The listing builds one solid part. Answer for the finished solid, in the listing's coordinates (mm). Round coordinates to 2 decimals unless told otherwise and drop trailing zeros. Loops run counter-clockwise (first coordinate to the right, second up) from the corner with the lowest first, then second, coordinate; pieces in that order, holes last. Notation, with made-up numbers: (10, 81.25) -> (32, 81.25) arc R23 cw to (32, 94.25) -> close; hole circle Ø9 at (41, 38). An arc over 180 degrees is marked (long way). Write each question's results on one line, items separated by ' | '. Start each with the question number.
from build123d import *

# Parameters (mm, degrees)
SKETCH_1_R      = 13.25
SKETCH_1_R_2    = 2
SKETCH_1_R_3    = 2.5
SKETCH_1_R_4    = 13
EXTRUDE_1_DEPTH = 5
FILLET_1_R      = 5


with BuildPart() as part:
    # 草图1 → 凸台-拉伸1 (new body)
    with BuildSketch(Plane.XY):
        with BuildLine():
            Line((0, 25), (124.869292101, 25))
            Line((124.869292101, 25), (184, 25))
            ThreePointArc((184, 25), (208.968890762, 1.246793543), (186.490484142, -24.875640469))
            Line((186.490484142, -24.875640469), (124.869292101, -25))
            Line((124.869292101, -25), (0, -25))
            Line((0, -25), (-16, -25))
            Line((-16, -25), (-16, 25))
            Line((-16, 25), (0, 25))
        make_face()
        with Locations((184, 0)):
            Circle(SKETCH_1_R, mode=Mode.SUBTRACT)
        with Locations((5, 16)):
            Circle(SKETCH_1_R_2, mode=Mode.SUBTRACT)
        with Locations(Location((5, -16, 0), (0, 0, 180))):
            Circle(SKETCH_1_R_2, mode=Mode.SUBTRACT)
        with Locations((60, 18)):
            Circle(SKETCH_1_R_3, mode=Mode.SUBTRACT)
        with Locations((124, 18)):
            Circle(SKETCH_1_R_3, mode=Mode.SUBTRACT)
        with Locations((34, 0)):
            Circle(SKETCH_1_R_4, mode=Mode.SUBTRACT)
        with Locations((34, 17.5)):
            Circle(SKETCH_1_R_2, mode=Mode.SUBTRACT)
        with Locations(Location((124, -18, 0), (0, 0, 180))):
            Circle(SKETCH_1_R_3, mode=Mode.SUBTRACT)
        with Locations(Location((60, -18, 0), (0, 0, 180))):
            Circle(SKETCH_1_R_3, mode=Mode.SUBTRACT)
        with Locations((51.5, 0)):
            Circle(SKETCH_1_R_2, mode=Mode.SUBTRACT)
        with Locations((34, -17.5)):
            Circle(SKETCH_1_R_2, mode=Mode.SUBTRACT)
        with Locations((16.5, 0)):
            Circle(SKETCH_1_R_2, mode=Mode.SUBTRACT)
        with Locations((-7, 16)):
            Circle(SKETCH_1_R_2, mode=Mode.SUBTRACT)
        with Locations(Location((-7, -16, 0), (0, 0, 180))):
            Circle(SKETCH_1_R_2, mode=Mode.SUBTRACT)
        with BuildLine():
            Line((75, -12), (110, -12))
            ThreePointArc((110, -12), (113, -9), (110, -6))
            Line((110, -6), (75, -6))
            ThreePointArc((75, -6), (72, -9), (75, -12))
        make_face(mode=Mode.SUBTRACT)
        with BuildLine():
            Line((124, 3), (159, 3))
            ThreePointArc((159, 3), (162, 0), (159, -3))
            Line((159, -3), (124, -3))
            ThreePointArc((124, -3), (121, 0), (124, 3))
        make_face(mode=Mode.SUBTRACT)
        with BuildLine():
            Line((75, 12), (110, 12))
            ThreePointArc((110, 12), (113, 9), (110, 6))
            Line((110, 6), (75, 6))
            ThreePointArc((75, 6), (72, 9), (75, 12))
        make_face(mode=Mode.SUBTRACT)
    extrude(amount=EXTRUDE_1_DEPTH)

    # 圆角1
    fillet_1_edges = [part.edges().sort_by_distance(p)[0] for p in [
        (-16, -25, 2.5),
        (-16, 25, 2.5),
    ]]
    fillet(fillet_1_edges, radius=FILLET_1_R)


solid = part.part
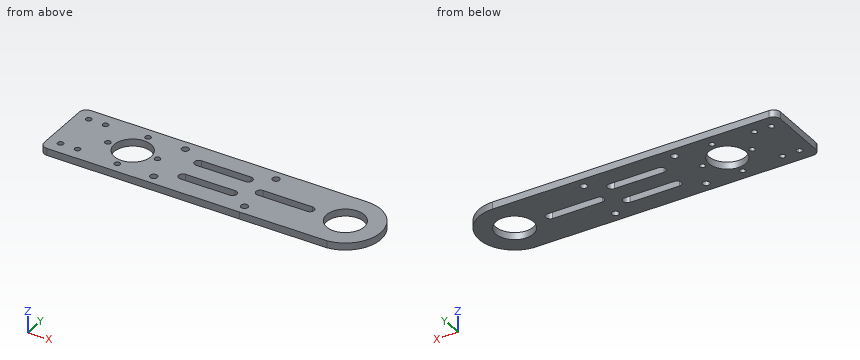
Item 1: The part is cut by section B-B, the plane x = 34. Give the vertices of the cut face in (y, z), plus the area to 3 significant figures.
Item 2: The part is cut by section A-A, the plane x = 5. Give the vertices of the cut face in (y, z), plus the area to 3 significant figures.
Item 3: Straight lines are drawn through the part: L1, parallel to Y at x = 5, z = 2; L2, parallel to Y at x = 110.5, z = 1.75; L3, parallel to X at y = 11, z = 1.95. For each, find the intervals that lie inside material, in ascending order. Write a range as [from, to].
Item 4: Each of these flat-tipped pins is pushed along its axis until it touches: pin 1 Ø3 at (x, z) = (139, 2) entering from -Y; pin 2 Ø2 at (y, z) = (-5, 1) entering from +X. Where does it stop, or does it pass through?
Item 5: The part is cut by section C-C, the plane y = 8.5. Give the vertices of the cut face in (x, z), plus the area to 3 significant figures.
Item 6: The part is cut by section D-D, the plane z = 3.2. Give the number of separate pieces and of enclosed holes in the cut face, plus the area to 3 significant figures.
Report:
1) outline: (-25, 0) -> (-19.5, 0) -> (-19.5, 5) -> (-25, 5) -> close; (-15.5, 0) -> (-13, 0) -> (-13, 5) -> (-15.5, 5) -> close; (13, 0) -> (15.5, 0) -> (15.5, 5) -> (13, 5) -> close; (19.5, 0) -> (25, 0) -> (25, 5) -> (19.5, 5) -> close | area: 80.0 mm2
2) outline: (-25, 0) -> (-18, 0) -> (-18, 5) -> (-25, 5) -> close; (-14, 0) -> (14, 0) -> (14, 5) -> (-14, 5) -> close; (18, 0) -> (25, 0) -> (25, 5) -> (18, 5) -> close | area: 210 mm2
3) L1: y = [-25, -18], [-14, 14], [18, 25] | L2: y = [-25, -11.96], [-6.04, 6.04], [11.96, 25] | L3: x = [-16, 27.07], [40.93, 72.76], [112.24, 176.61], [191.39, 206.45]
4) pin 1: stops at y = -24.97 | pin 2: stops at x = 208.68
5) outline: (-16, 0) -> (24.16, 0) -> (24.16, 5) -> (-16, 5) -> close; (43.84, 0) -> (72.04, 0) -> (72.04, 5) -> (43.84, 5) -> close; (112.96, 0) -> (173.84, 0) -> (173.84, 5) -> (112.96, 5) -> close; (194.16, 0) -> (207.51, 0) -> (207.51, 5) -> (194.16, 5) -> close | area: 713 mm2
6) separate pieces: 1 | enclosed holes: 17 | area: 8,990 mm2
